The listing builds one solid part. Answer for the finished solid, in the listing's coordinates (mm). Give positions to 0.01 mm unless a question says otherwise; leave off trailing zeros. Write each loop counter-clockwise with the first axis right and the second up, starting at its lowest first coordinate (ties: lowest second). Pieces come first, ordered by that corner, then holes. Notation, with made-up numbers: (89, -38) - (137, -38) arc R5 ccw to (137, -34) - close; hole circle Ø1 at (47.5, 14). An arc over 180 degrees is marked (long way). Use a Markdown table: item, result. Add a question column.
from build123d import *

# Parameters (mm, degrees)
F0_W     = 40
F0_H     = 49
F1_DEPTH = 20
F3_D     = 7
F3_DEPTH = 23
F3_TIP   = 2.1030121666


with BuildPart() as f1:
    # F0 (on Top) → F1 (new body)
    with BuildSketch(Plane.XY):
        Rectangle(F0_W, F0_H)
    extrude(amount=-F1_DEPTH)

    # F3
    with Locations(Plane.XY):
        with Locations((0, -12.5), (0, 12.5)):
            Hole(F3_D / 2, depth=F3_DEPTH)
            with Locations((0, 0, -(F3_DEPTH + F3_TIP / 2))):  # 118° drill point
                Cone(0, F3_D / 2, F3_TIP, mode=Mode.SUBTRACT)


solid = f1.part
1. The part is cut by section C-C (x = 0). Give the vertices of the cut face in (y, z), and give its area (3 significant figures).
2. For a pull along Y with two mould halves and no side action, classify faces 1 (the flat face through (-20, 0, -10)), 2 (the cylindrical face through (0.759, -15.917, -10.14)), 3 (the flat face through (0, 24.5, -10)), 4 (the cylindrical face through (0.759, 9.083, -10.14)) as released by +Y, released by -Y, zero draft, split by the parting line, or undercut.
3. Given P1, Ø11, axis at x = 0, y = 12.5, coming from the +Z side, flat-ended and moving along its own axis, determine where the tip first touches the part or whether it passes through.
4. Consider L1, parallel to Y at x = 0, z = -10.25; L2, parallel to Y at x = -1.5, z = -11.25; L3, parallel to X at y = -15.5, z = -5. Determine where each line is inside the solid, lowest interval first. Write a range as [from, to].
5. The part is cut by section B-B (z = -5). Give the vertices of the cut face in (x, y).
6. The part is cut by section A-A (y = -12.5). Give the vertices of the cut face in (x, z), and give its area (3 significant figures).
Check values:
| question | item | result |
|---|---|---|
| 1 | outline | (-24.5, -20) - (-16, -20) - (-16, 0) - (-24.5, 0) - close; (-9, -20) - (9, -20) - (9, 0) - (-9, 0) - close; (16, -20) - (24.5, -20) - (24.5, 0) - (16, 0) - close |
| 1 | area | 700 mm2 |
| 2 | face 1 | zero draft |
| 2 | face 2 | undercut |
| 2 | face 3 | released by +Y |
| 2 | face 4 | undercut |
| 3 | P1 | stops at z = 0 |
| 4 | L1 | y = [-24.5, -16], [-9, 9], [16, 24.5] |
| 4 | L2 | y = [-24.5, -15.66], [-9.34, 9.34], [15.66, 24.5] |
| 4 | L3 | x = [-20, -1.8], [1.8, 20] |
| 5 | outline | (-20, -24.5) - (20, -24.5) - (20, 24.5) - (-20, 24.5) - close; hole circle Ø7 at (0, -12.5); hole circle Ø7 at (0, 12.5) |
| 6 | outline | (-20, -20) - (-3.5, -20) - (-3.5, 0) - (-20, 0) - close; (3.5, -20) - (20, -20) - (20, 0) - (3.5, 0) - close |
| 6 | area | 660 mm2 |
